Autodesk Inventor part; units mm, degrees
ref_plane "YZ Plane" through (0, 0, 0) normal (1, 0, 0) x (0, 1, 0)
ref_plane "XZ Plane" through (0, 0, 0) normal (0, 1, 0) x (-1, 0, 0)
ref_plane "XY Plane" through (0, 0, 0) normal (0, 0, 1) x (1, 0, 0)
sketch "Sketch1" plane through (0, 0, 0) normal (0, 0, 1) x (1, 0, 0)
  line L0 (50.75, 32.3006) -> (46.25, 32.3006)
  line L1 (46.25, 32.3006) -> (46.25, 39.8006)
  line L2 (46.25, 39.8006) -> (50.75, 39.8006)
  arc A0 (50.75, 39.8006) -> (56.25, 45.3006) centre (50.75, 45.3006) ccw
  line L3 (56.25, 45.3006) -> (56.25, 49.8006)
  line L4 (56.25, 49.8006) -> (63.75, 49.8006)
  line L5 (63.75, 49.8006) -> (63.75, 45.3006)
  arc A1 (63.75, 45.3006) -> (69.2516, 39.8006) centre (69.25, 45.3006) ccw
  line L6 (69.2516, 39.8006) -> (73.7503, 39.8165)
  line L7 (73.7503, 39.8165) -> (73.7589, 32.3006)
  line L8 (73.7589, 32.3006) -> (69.25, 32.3006)
  arc A2 (69.25, 32.3006) -> (63.75, 26.8006) centre (69.25, 26.8006) ccw
  line L9 (63.75, 26.8006) -> (63.75, 22.3006)
  line L10 (63.75, 22.3006) -> (56.25, 22.3006)
  line L11 (56.25, 22.3006) -> (56.25, 26.8006)
  arc A3 (56.25, 26.8006) -> (50.75, 32.3006) centre (50.75, 26.8006) ccw
  line L12 (47.25, 33.3006) -> (50.75, 33.3006)
  arc A4 (57.25, 26.8006) -> (50.75, 33.3006) centre (50.75, 26.8006) ccw
  line L13 (57.25, 26.8006) -> (57.25, 23.3006)
  line L14 (57.25, 23.3006) -> (62.75, 23.3006)
  line L15 (62.75, 23.3006) -> (62.75, 26.8006)
  arc A5 (69.25, 33.3006) -> (62.75, 26.8006) centre (69.25, 26.8006) ccw
  line L16 (69.25, 33.3006) -> (72.7578, 33.3006)
  line L17 (72.7578, 33.3006) -> (72.7514, 38.813)
  line L18 (72.7514, 38.813) -> (69.2535, 38.8006)
  arc A6 (62.75, 45.3006) -> (69.2535, 38.8006) centre (69.25, 45.3006) ccw
  line L19 (62.75, 45.3006) -> (62.75, 48.8006)
  line L20 (62.75, 48.8006) -> (57.25, 48.8006)
  line L21 (57.25, 48.8006) -> (57.25, 45.3006)
  arc A7 (50.75, 38.8006) -> (57.25, 45.3006) centre (50.75, 45.3006) ccw
  line L22 (50.75, 38.8006) -> (47.25, 38.8006)
  line L23 (47.25, 38.8006) -> (47.25, 33.3006)
  point P0 (0, 0)
  dimension "d47" = 1
extrude "Extrusion1" add sketch "Sketch1" along normal blind 6 contours L0 L1 L2 A0 L3 L4 L5 A1 L6 L7 L8 A2 L9 L10 L11 A3 | L23 L22 A7 L21 L20 L19 A6 L18 L17 L16 A5 L15 L14 L13 A4 L12
sketch "Sketch2" plane through (0, 0, 6) normal (0, 0, 1) x (1, 0, 0)
  line L0 (50.75, 32.3006) -> (46.25, 32.3006)
  line L1 (46.25, 32.3006) -> (46.25, 39.8006)
  line L2 (46.25, 39.8006) -> (50.75, 39.8006)
  arc A0 (50.75, 39.8006) -> (56.25, 45.3006) centre (50.75, 45.3006) ccw
  line L3 (56.25, 49.8006) -> (63.75, 49.8006)
  line L4 (63.75, 49.8006) -> (63.75, 45.3006)
  arc A1 (63.75, 45.3006) -> (69.2516, 39.8006) centre (69.25, 45.3006) ccw
  line L5 (69.2516, 39.8006) -> (73.7498, 39.8006)
  line L6 (73.7498, 39.8006) -> (73.732, 32.3006)
  line L7 (73.732, 32.3006) -> (69.25, 32.3006)
  arc A2 (69.25, 32.3006) -> (63.75, 26.8006) centre (69.25, 26.8006) ccw
  line L8 (63.75, 26.8006) -> (63.75, 22.3006)
  line L9 (63.75, 22.3006) -> (56.25, 22.3006)
  line L10 (56.25, 22.3006) -> (56.25, 26.8006)
  arc A3 (56.25, 26.8006) -> (50.75, 32.3006) centre (50.75, 26.8006) ccw
  line L11 (47.25, 33.3006) -> (50.75, 33.3006)
  arc A4 (57.25, 26.8006) -> (50.75, 33.3006) centre (50.75, 26.8006) ccw
  line L12 (57.25, 26.8006) -> (57.25, 23.3006)
  line L13 (57.25, 23.3006) -> (62.75, 23.3006)
  line L14 (62.75, 23.3006) -> (62.75, 26.8006)
  arc A5 (69.25, 33.3006) -> (62.75, 26.8006) centre (69.25, 26.8006) ccw
  line L15 (69.25, 33.3006) -> (72.7343, 33.3006)
  line L16 (72.7343, 33.3006) -> (72.7474, 38.8006)
  line L17 (72.7474, 38.8006) -> (69.2516, 38.8006)
  arc A6 (62.75, 45.3006) -> (69.2516, 38.8006) centre (69.25, 45.3006) ccw
  line L18 (62.75, 45.3006) -> (62.75, 48.8006)
  line L19 (62.75, 48.8006) -> (57.25, 48.8006)
  line L20 (57.25, 48.8006) -> (57.25, 45.3006)
  arc A7 (50.75, 38.8006) -> (57.25, 45.3006) centre (50.75, 45.3006) ccw
  line L21 (50.75, 38.8006) -> (47.25, 38.8006)
  line L22 (47.25, 38.8006) -> (47.25, 33.3006)
  line L23 (50.75, 33.3006) -> (50.75, 32.3006)
  line L24 (50.75, 38.8006) -> (50.75, 39.8006)
  line L25 (56.25, 49.8006) -> (56.25, 45.3006)
  line L26 (56.25, 45.3006) -> (57.25, 45.3006)
  line L27 (62.75, 45.3006) -> (63.75, 45.3006)
  line L28 (69.2516, 38.8006) -> (69.2516, 39.8006)
  line L29 (69.25, 33.3006) -> (69.25, 32.3006)
  line L30 (62.75, 26.8006) -> (63.75, 26.8006)
  line L31 (56.25, 26.8006) -> (56.25, 22.3006)
  line L32 (56.25, 26.8006) -> (57.25, 26.8006)
  dimension "d48" = 1
sketch "Sketch4" plane through (0, 0, 0) normal (0, 0, -1) x (-1, 0, 0)
  line L0 (-73.75, 32.3006) -> (-73.75, 39.8006)
  line L1 (-73.75, 36.0506) -> (-46.25, 36.0506)
  line L2 (-46.25, 39.8006) -> (-46.25, 32.3006)
  circle A0 centre (-60, 36.0506) radius 3
  point P0 (0, 0)
  dimension "d31" = 6
extrude "Extrusion4" add sketch "Sketch4" along normal blind 2.7
fillet "Fillet4" radius 2 1 edges at (63, 36.0506, -2.7)
extrude "Extrusion7" cut sketch "Sketch2" against normal blind 4.6 contours L23 A4 L32 A3 | A0 L26 A7 L24 | L30 A5 L29 A2 | A1 L28 A6 L27
sketch "Sketch5" plane through (0, 0, 6) normal (0, 0, 1) x (1, 0, 0)
  line L0 (62.75, 23.3006) -> (62.75, 26.8006)
  line L1 (63.75, 26.8006) -> (63.75, 22.3006)
  line L2 (57.25, 26.8006) -> (57.25, 23.3006)
  line L3 (57.25, 23.3006) -> (62.75, 23.3006)
  line L4 (56.25, 22.3006) -> (56.25, 26.8006)
  line L5 (63.75, 22.3006) -> (56.25, 22.3006)
  line L6 (56.25, 49.8006) -> (63.75, 49.8006)
  line L7 (63.75, 49.8006) -> (63.75, 45.3006)
  line L8 (57.25, 48.8006) -> (57.25, 45.3006)
  line L9 (62.75, 48.8006) -> (57.25, 48.8006)
  line L10 (62.75, 45.3006) -> (62.75, 48.8006)
  line L11 (50.75, 32.3006) -> (46.25, 32.3006)
  line L12 (46.25, 32.3006) -> (46.25, 39.8006)
  line L13 (46.25, 39.8006) -> (50.75, 39.8006)
  line L14 (47.25, 33.3006) -> (50.75, 33.3006)
  line L15 (47.25, 38.8006) -> (47.25, 33.3006)
  line L16 (50.75, 38.8006) -> (47.25, 38.8006)
  line L17 (50.75, 33.3006) -> (50.75, 32.3006)
  line L18 (50.75, 38.8006) -> (50.75, 39.8006)
  line L19 (56.25, 49.8006) -> (56.25, 45.3006)
  line L20 (56.25, 45.3006) -> (57.25, 45.3006)
  line L21 (62.75, 45.3006) -> (63.75, 45.3006)
  line L22 (62.75, 26.8006) -> (63.75, 26.8006)
  line L23 (56.25, 26.8006) -> (56.25, 22.3006)
  line L24 (56.25, 26.8006) -> (57.25, 26.8006)
  line L25 (73.7589, 32.3006) -> (69.25, 32.3006)
  line L26 (69.25, 32.3006) -> (73.7589, 32.3006)
  line L27 (73.7589, 32.3006) -> (73.7503, 39.8165)
  line L28 (73.7589, 32.3006) -> (73.7503, 39.8165)
  line L29 (69.2516, 39.8006) -> (73.7503, 39.8165)
  line L30 (73.7503, 39.8165) -> (69.2516, 39.8006)
  line L31 (69.2516, 39.8006) -> (69.2516, 38.8006)
  line L32 (69.2516, 39.8006) -> (69.2516, 38.8006)
  line L33 (69.25, 33.3006) -> (69.25, 32.3006)
  line L34 (69.25, 32.3006) -> (69.25, 33.3006)
  line L35 (69.25, 33.3006) -> (72.7582, 33.3006)
  line L36 (72.7582, 33.3006) -> (72.7582, 38.8006)
  line L37 (72.7582, 38.8006) -> (69.2516, 38.8006)
  point P0 (0, 0)
  point P1 (50.75, 26.8006)
  dimension "d51" = 1
extrude "Extrusion8" cut sketch "Sketch5" against normal blind 6
fillet "Fillet6" radius 1 8 edges at (72.7582, 33.3006, 3) (72.7582, 38.8006, 3) (62.75, 23.3006, 3) (57.25, 23.3006, 3) (62.75, 48.8006, 3) (57.25, 48.8006, 3) (47.25, 38.8006, 3) (47.25, 33.3006, 3)
fillet "Fillet7" radius 1 8 edges at (69.25, 32.3006, 0.7) (63.75, 26.8006, 0.7) (69.2516, 39.8006, 0.7) (63.75, 45.3006, 0.7) (56.25, 26.8006, 0.7) (50.75, 32.3006, 0.7) (56.25, 45.3006, 0.7) (50.75, 39.8006, 0.7)
properties part number "Groboy Buttons D-Pad"
Model file for the job. Use its own axes, mm. A direction names the side the tool comes from. Coordinates: 2 decimals unless noted, no trailing zeros. Loops run counter-clockwise (first coordinate to the right, second up) from the corner with the lowest first, then second, coordinate; pieces in that order, holes last. Notation, with made-up numbers: (45, -0.5) - (68, -0.5) arc R30 ccw to (68, 26.5) - close; hole circle Ø1 at (6.5, 0). An arc over 180 degrees is marked (long way). Answer as a JSON object with one key per item and string values. Group by question number.
(1) Flat gauge pins, fed straight in: pin 1 (1.3 mm diameter, centred on x = 70, z = 4, fed in from -Y); pin 2 (2 mm diameter, centred on y = 25, z = 4.5, fed in from +X); pin 3 (12 mm diameter, centred on x = 67.5, y = 34, fed in from -Z). Where does each tip first touch, or does it go through?
(2) Tool access for faces 1 (the face through (57.25, 26, 3)), 2 (the face through (70, 33.301, 3)), 3 (the face through (62.75, 47, 3)): list every direction of +Z, -Z, +X, -X, +Y, -Y with a clear straight run to the whole face (end or side of a thin tool).
(3) Two-plate mould, pull along Z, no slides. Class faces 4 (the face through (60, 36, 6)), 5 (the face through (57.25, 47, 3)), 6 (the face through (63, 33, 0)): released by +Z, released by -Z, zero draft, split by the parting line, or undercut.
(4) Cut at A-A (z = 3). Give the cut face in (x, y), then the cut area to 3 significant figures.
(5) Cut at C-C (x = 67). Give the cut face in (y, z), then the cut area to 3 significant figures.
(6) Probe line 1 along Z through (x, y) = (55.75, 32.75); line 2 along X through (y, z) = (26, 1.25); line 3 along Y through (x, z) = (53.5, 5.25). List the from-to ranges inside material, lowest first.
(7) Cut at D-D (x = 52.75). Give the cut face in (y, z).
(8) Cut at B-B (x = 70). Give the cut face in (y, z), then the cut area to 3 significant figures.
Geometry says:
{
 "1": {"pin 1": "stops at y = 33.3", "pin 2": "stops at x = 62.75", "pin 3": "stops at z = -2.54"},
 "2": {"face 1": "+Z, -Z, -X, -Y", "face 2": "+Z, -Z, +X, -Y", "face 3": "+Z, -Z, +X, +Y"},
 "3": {"face 4": "released by +Z", "face 5": "zero draft", "face 6": "released by -Z"},
 "4": {"outline": "(47.25, 34.3) arc R1 ccw to (48.25, 33.3) - (50.75, 33.3) arc R6.5 cw to (57.25, 26.8) - (57.25, 24.3) arc R1 ccw to (58.25, 23.3) - (61.75, 23.3) arc R1 ccw to (62.75, 24.3) - (62.75, 26.8) arc R6.5 cw to (69.25, 33.3) - (71.76, 33.3) arc R1 ccw to (72.76, 34.3) - (72.76, 37.8) arc R1 ccw to (71.76, 38.8) - (69.25, 38.8) arc R6.5 cw to (62.75, 45.3) - (62.75, 47.8) arc R1 ccw to (61.75, 48.8) - (58.25, 48.8) arc R1 ccw to (57.25, 47.8) - (57.25, 45.3) arc R6.5 cw to (50.75, 38.8) - (48.25, 38.8) arc R1 ccw to (47.25, 37.8) - close", "area": "285 mm^2"},
 "5": {"outline": "(31.82, 0) - (40.28, 0) - (40.28, 1.4) - (39.2, 1.4) - (39.2, 6) - (32.9, 6) - (32.9, 1.4) - (31.82, 1.4) - close", "area": "40.8 mm^2"},
 "6": {"line 1": "z = 0 to 6", "line 2": "x = 57.25 to 62.75", "line 3": "y = 32.69 to 39.41"},
 "7": {"outline": "(31.92, 0) - (40.18, 0) - (40.18, 1.4) - (39.12, 1.4) - (39.12, 6) - (32.99, 6) - (32.99, 1.4) - (31.92, 1.4) - close"},
 "8": {"outline": "(33.3, 0) - (38.8, 0) - (38.8, 6) - (33.3, 6) - close", "area": "33.0 mm^2"}
}
